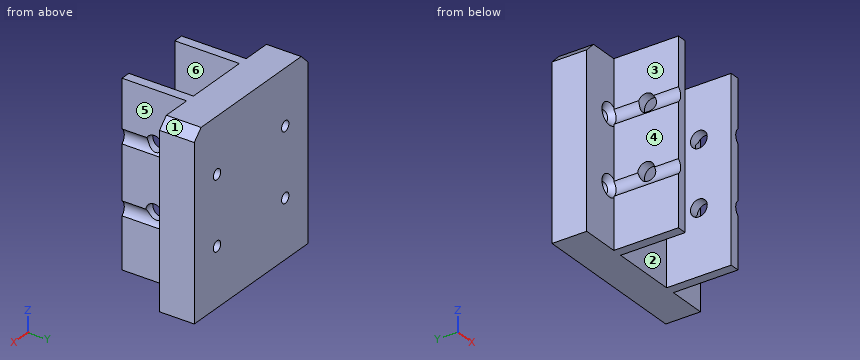
```python
from build123d import *

# Parameters (mm, degrees)
EXTRUDE_1_DEPTH             = 53
HOLE_WIZARD_1_D             = 3
SKETCH_6_R                  = 2.9
CUT_EXTRUDE_1_DEPTH         = 62.919302322
CHAMFER_1_SIZE              = 3
HOLE_WIZARD_2_D             = 5.2
HOLE_WIZARD_M3_1_AT_2_COUNT = 2
HOLE_WIZARD_M3_1_AT_2_PITCH = 30
HOLE_WIZARD_M3_1_AT_3_COUNT = 2
HOLE_WIZARD_M3_1_AT_3_PITCH = 36.619666847
HOLE_WIZARD_M3_1_AT_4_COUNT = 2
HOLE_WIZARD_M3_1_AT_4_PITCH = 21
EXTRUDE_2_DEPTH             = 3


with BuildPart() as part:
    # 草图1 → 凸台-拉伸1 (new body)
    with BuildSketch(Plane.XY):
        Polygon((-13.1, -14.961364275), (-10.1, -14.961364275), (-10.1, 5.038635725), (10.1, 5.038635725), (10.1, -14.961364275), (13.1, -14.961364275), (13.1, 5.038635725), (25, 5.038635725), (25, 15.788635725), (-25, 15.788635725), (-25, 5.038635725), (-13.1, 5.038635725), align=None)
    extrude(amount=EXTRUDE_1_DEPTH)

    # 孔1 (through all)
    with Locations(Plane(origin=(0, 5.038635725, 0), x_dir=(-1, 0, 0), z_dir=(0, -1, 0))):
        with Locations((15, -15), (15, -36), (-15, -15), (-15, -36)):
            Hole(HOLE_WIZARD_1_D / 2)

    # 草图6 → 切除-拉伸1 (cut, through all)
    with BuildSketch(Plane.XZ.offset(-5.038635725)):
        with Locations((15, 36)):
            Circle(SKETCH_6_R)
        with Locations((15, 15)):
            Circle(SKETCH_6_R)
        with Locations((-15, 15)):
            Circle(SKETCH_6_R)
        with Locations((-15, 36)):
            Circle(SKETCH_6_R)
    extrude(amount=CUT_EXTRUDE_1_DEPTH, mode=Mode.SUBTRACT)

    # 倒角1
    chamfer_1_edges = [part.edges().sort_by_distance(p)[0] for p in [
        (-25, 10.413635725, 53),
        (25, 10.413635725, 53),
    ]]
    chamfer(chamfer_1_edges, length=CHAMFER_1_SIZE)

    # 孔2 (through all)
    with Locations(Plane(origin=(13.1, 0, 0), x_dir=(0, 0, -1), z_dir=(1, 0, 0))):
        with Locations((-17, -4.961364275), (-37, -4.961364275)):
            Hole(HOLE_WIZARD_2_D / 2)

    # 草图10 → M3 十字槽沉头木螺钉的锥形沉头孔1 (revolve, cut)
    with BuildSketch(Plane(origin=(15, 5.038635725, 15), x_dir=(0, 0, -1), z_dir=(1, 0, 0))):
        Polygon((0, 0), (0, 10.75), (1.6, 10.75), (1.6, 1.7), (3.3, 0), align=None)
    hole_wizard_m3_1 = revolve(axis=Axis((15, -1.311364275, 15), (0, 1, 0)), mode=Mode.SUBTRACT)

    # M3 十字槽沉头木螺钉的锥形沉头孔1 at 2: M3 十字槽沉头木螺钉的锥形沉头孔1 ×2
    with Locations(*[(-i * HOLE_WIZARD_M3_1_AT_2_PITCH, 0, 0) for i in range(1, HOLE_WIZARD_M3_1_AT_2_COUNT)]):
        add(hole_wizard_m3_1, mode=Mode.SUBTRACT)

    # M3 十字槽沉头木螺钉的锥形沉头孔1 at 3: M3 十字槽沉头木螺钉的锥形沉头孔1 ×2
    with Locations(*[Vector(-0.8192319205190406, 0, 0.5734623443633283) * (i * HOLE_WIZARD_M3_1_AT_3_PITCH) for i in range(1, HOLE_WIZARD_M3_1_AT_3_COUNT)]):
        add(hole_wizard_m3_1, mode=Mode.SUBTRACT)

    # M3 十字槽沉头木螺钉的锥形沉头孔1 at 4: M3 十字槽沉头木螺钉的锥形沉头孔1 ×2
    with Locations(*[(0, 0, i * HOLE_WIZARD_M3_1_AT_4_PITCH) for i in range(1, HOLE_WIZARD_M3_1_AT_4_COUNT)]):
        add(hole_wizard_m3_1, mode=Mode.SUBTRACT)

    # 草图12 → 凸台-拉伸2 (add)
    with BuildSketch(Plane(origin=(0, 0, 0), x_dir=(-1, 0, 0), z_dir=(0, 0, -1))):
        Polygon((-10.1, 5.038635725), (10.1, 5.038635725), (10.1, -14.961364275), (13.1, -14.961364275), (13.1, 5.038635725), (25, 5.038635725), (25, 15.788635725), (-25, 15.788635725), (-25, 5.038635725), (-13.1, 5.038635725), (-13.1, -14.961364275), (-10.1, -14.961364275), align=None)
    extrude(amount=EXTRUDE_2_DEPTH)


solid = part.part
```
The listing builds one solid part. Answer for the finished solid, in the listing's coordinates (mm). Face numbers are marked on the shaded views. A direction names the side the tool comes from. Give positions to 0.01 mm unless a question says otherwise; leave off trailing zeros. Write each loop counter-clockwise with the first axis right and the second up, starting at its lowest first coordinate (ties: lowest second). Pieces come first, ordered by that corner, then holes. Notation, with made-up numbers: (61, 43.5) - (90, 43.5) arc R21 ccw to (90, 66.5) - close; hole circle Ø5 at (63, 46). An arc over 180 degrees is marked (long way). Use one line per item in the form item = value. Start each with the question number.
1) Find section A-A on x = 15. Determine the outline of the cut face in (y, z), plus the area to 3 significant figures.
2) The mould has two halves that part along X. Classify the marked faces 1, 2 and 3: pulls with the +X half, pulls with the -X half, needs draft (parallel to the pull), parting line crosses it, or undercut.
3) Flat-ended cylindrical pins translate along their axes: pin 1 Ø4 at (x, z) = (15, 15) entering from -Y; pin 2 Ø10 at (x, z) = (3, 26.5) entering from -Y; pin 3 Ø17.5 at (y, z) = (-9, 8.5) entering from +X; pin 4 Ø10 at (x, y) = (17.5, 2.5) entering from +Z. Find the tip coordinate at first contact, or state that the pin passes through.
4) Consider line 1 along Z through (x, y) = (15, 13); line 2 along X through (y, z) = (9, 15); line 3 along X through (y, z) = (2, 17.5). Determine where each line is inside the solid, lowest interval first. Write a range as from..to.
5) Find section D-D on z = 36. Count the separate pieces of the cut face and the enclosed holes in it, plus the area to 3 significant figures.
6) Find section B-B on y = -1.5. Determine the outline of the cut face in (x, z), plus the area to 3 significant figures.
7) A tool of negligible diameter and unlimited length cuts with its end or side. For the marked faces 4, 5 and 6, from which of +Z, -Z, +X, -X, +Y, -Y can it reach the whole face along a straight path? Write none if from no direction.
8) Find section C-C on z = 23. Determine the outline of the cut face in (x, y), plus the area to 4 significant figures.
Geometry results:
q1.outline = (5.04, -3) - (15.79, -3) - (15.79, 13.4) - (6.74, 13.4) - (5.04, 11.7) - close; (5.04, 18.3) - (6.74, 16.6) - (15.79, 16.6) - (15.79, 34.4) - (6.74, 34.4) - (5.04, 32.7) - close; (5.04, 39.3) - (6.74, 37.6) - (15.79, 37.6) - (15.79, 53) - (5.04, 53) - close
q1.area = 527 mm2
q2.face_1 = pulls with the +X half
q2.face_2 = undercut
q2.face_3 = pulls with the -X half
q3.pin_1 = 6.34
q3.pin_2 = 5.04
q3.pin_3 = 13.1
q3.pin_4 = 53
q4.line_1 = -3..13.4, 16.6..34.4, 37.6..53
q4.line_2 = -25..-16.6, -13.4..13.4, 16.6..25
q4.line_3 = -13.1..-10.1, 10.1..13.1
q5.separate_pieces = 5
q5.enclosed_holes = 0
q5.area = 524 mm2
q6.outline = (-13.1, -3) - (-10.1, -3) - (-10.1, 53) - (-13.1, 53) - (-13.1, 38.19) arc R2.9 cw to (-13.1, 33.81) - (-13.1, 17.19) arc R2.9 cw to (-13.1, 12.81) - close; (10.1, -3) - (13.1, -3) - (13.1, 12.81) arc R2.9 cw to (13.1, 17.19) - (13.1, 33.81) arc R2.9 cw to (13.1, 38.19) - (13.1, 53) - (10.1, 53) - close
q6.area = 324 mm2
q7.face_4 = +Z, -Z, -X, -Y
q7.face_5 = +Z, -Z, +X, -Y
q7.face_6 = +Z, -Z, -Y
q8.outline = (-25, 5.04) - (-13.1, 5.04) - (-13.1, -14.96) - (-10.1, -14.96) - (-10.1, 5.04) - (10.1, 5.04) - (10.1, -14.96) - (13.1, -14.96) - (13.1, 5.04) - (25, 5.04) - (25, 15.79) - (-25, 15.79) - close
q8.area = 657.5 mm2
